For this review, take the finished solid that the model builds, in its own axes (mm). Face numbers are marked on the shaded views. A direction names the side the tool comes from. Coordinates: 2 decimals unless noted, no trailing zeros. Loops run counter-clockwise (first coordinate to the right, second up) from the corner with the lowest first, then second, coordinate; pieces in that order, holes last. Notation, with made-up numbers: M 15,66 L 27,66 A36 cw 27,101 Z; hole C -36.75,-37 d1. An arc over 180 degrees is marked long. Put each result on its own line as item: value.
```python
from build123d import *

# Parameters (mm, degrees)
SKETCH1_W           = 30
SKETCH1_H           = 20
BOSS_EXTRUDE1_DEPTH = 10
SKETCH3_W           = 12.55
SKETCH3_H           = 20
BOSS_EXTRUDE3_DEPTH = 20
SKETCH6_R           = 2.3
CUT_EXTRUDE1_DEPTH  = 33.015621187
SKETCH7_R           = 1.625
CUT_EXTRUDE2_DEPTH  = 141.678400141


with BuildPart() as part:
    # Sketch1 → Boss-Extrude1 (new body)
    with BuildSketch(Plane(origin=(0, 0, 0), x_dir=(1, 0, 0), z_dir=(0, 1, 0))):
        Rectangle(SKETCH1_W, SKETCH1_H)
    extrude(amount=BOSS_EXTRUDE1_DEPTH)

    # Sketch3 → Boss-Extrude3 (add)
    with BuildSketch(Plane.XZ):
        with Locations((8.725, 0)):
            Rectangle(SKETCH3_W, SKETCH3_H)
        with Locations((-8.725, 0)):
            Rectangle(SKETCH3_W, SKETCH3_H)
    extrude(amount=BOSS_EXTRUDE3_DEPTH)

    # Sketch6 → Cut-Extrude1 (cut, through all)
    with BuildSketch(Plane(origin=(0, 0, -10), x_dir=(-1, 0, 0), z_dir=(0, 0, -1))):
        with Locations((8, 5)):
            Circle(SKETCH6_R)
        with Locations((-8, 5)):
            Circle(SKETCH6_R)
    extrude(amount=-CUT_EXTRUDE1_DEPTH, mode=Mode.SUBTRACT)

    # Sketch7 → Cut-Extrude2 (cut, through all)
    with BuildSketch(Plane(origin=(-15, -86.420292381, -87.946615477), x_dir=(0, 1, 0), z_dir=(-1, 0, 0))):
        with Locations(Location((76.454314497, -88.455505565, 0), (0, 0, 270))):
            Circle(SKETCH7_R)
    extrude(amount=-CUT_EXTRUDE2_DEPTH, mode=Mode.SUBTRACT)


solid = part.part
```
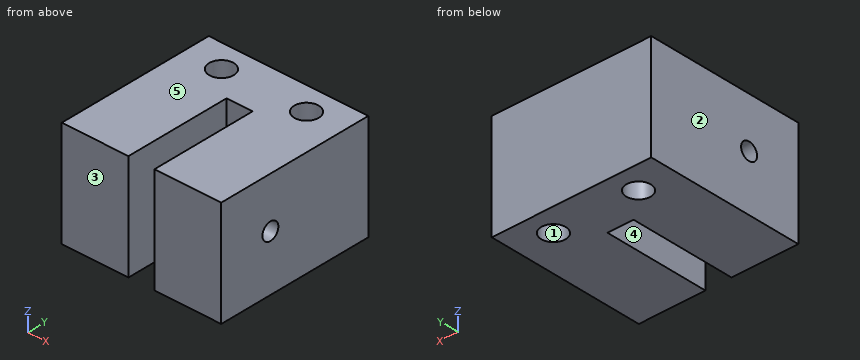
(1) Add section C-C (y = 5). Write out the cut boundary in (x, z).
Determined:
outline: M -15,-10 L -10.3,-10 L -10.3,10 L -15,10 Z; M -5.7,-10 L 5.7,-10 L 5.7,10 L -5.7,10 Z; M 10.3,-10 L 15,-10 L 15,10 L 10.3,10 Z
(2) Add section D-D (x = -7.25). Write out the cut boundary in (y, z) (3 decimals), plus the area to 3 significant figures.
Determined:
outline: M -20,-10 L 2.826,-10 L 2.826,10 L -20,10 Z; M 7.174,-10 L 10,-10 L 10,10 L 7.174,10 Z; hole C -9.966,0.509 d3.25
area: 505 mm^2
(3) Add section B-B (y = -4.75). Write out the cut boundary in (x, z), plus the area to 3 significant figures.
Determined:
outline: M -15,-10 L -2.45,-10 L -2.45,10 L -15,10 Z; M 2.45,-10 L 15,-10 L 15,10 L 2.45,10 Z
area: 502 mm^2
(4) For pin 1 (3 mm diameter, centred on x = 8, y = 5, fed in from +Z); pin 2 (1.5 mm diameter, centred on x = 0, z = -0.5, fed in from -Y), all flat-tipped, find the tip position at first contact; note any pin that passes through.
Determined:
pin 1: passes through
pin 2: stops at y = 0
(5) Draft analysis for pull direction X (two halves, no side actions). For the marked faces 1, 2 and 3, state which applies: +X half, -X half, draft (parallel to the pull), parting line (faces both ways), or undercut.
Determined:
face 1: undercut
face 2: -X half
face 3: draft
(6) Add section A-A (z = 0.5). Write out the cut boundary in (x, y), plus the area to 3 significant figures.
Determined:
outline: M -15,-20 L -2.45,-20 L -2.45,-11.59 L -15,-11.59 Z; M -15,-8.34 L -2.45,-8.34 L -2.45,0 L 2.45,0 L 2.45,-8.34 L 15,-8.34 L 15,10 L -15,10 Z; M 2.45,-20 L 15,-20 L 15,-11.59 L 2.45,-11.59 Z; hole C -8,5 d4.6; hole C 8,5 d4.6
area: 687 mm^2
(7) Wall thickness on line 1 along X through (y, z) = (-13, -4.75); line 2 along Y through (x, z) = (-9.75, 2); line 3 along X through (y, z) = (3.75, -2.5): over which ranges is each line inside the solid? List them lowest first. Write a range as [from, to].
Determined:
line 1: x = [-15, -2.45], [2.45, 15]
line 2: y = [-20, -10.61], [-9.32, 3.51], [6.49, 10]
line 3: x = [-15, -9.93], [-6.07, 6.07], [9.93, 15]
(8) Tool access review of the marked faces 4 and 5: name each direction out of +Z, -Z, +X, -X, +Y, -Y from which nothing blocks a thin tool from reaching the whole face with its end or side.
Determined:
face 4: +Z, -Z, -Y
face 5: +Z, +X, -X, +Y, -Y
